Drawing for the job (mm, zero at the part's lowest x, y, z). Coordinates: 2 decimals unless noted, no trailing zeros. Write each loop counter-clockwise with the first axis right and the second up, starting at its lowest first coordinate (ties: lowest second). Pieces come first, ordered by that corner, then holes. Notation, with made-up numbers: M 11.25,67.25 L 29.25,67.25 A24 cw 29.25,84.25 Z; hole C 49,77 d2. An arc over 180 degrees is marked long. Use CSV: the item, a comma, the result in double quotes. Start each with the question number.
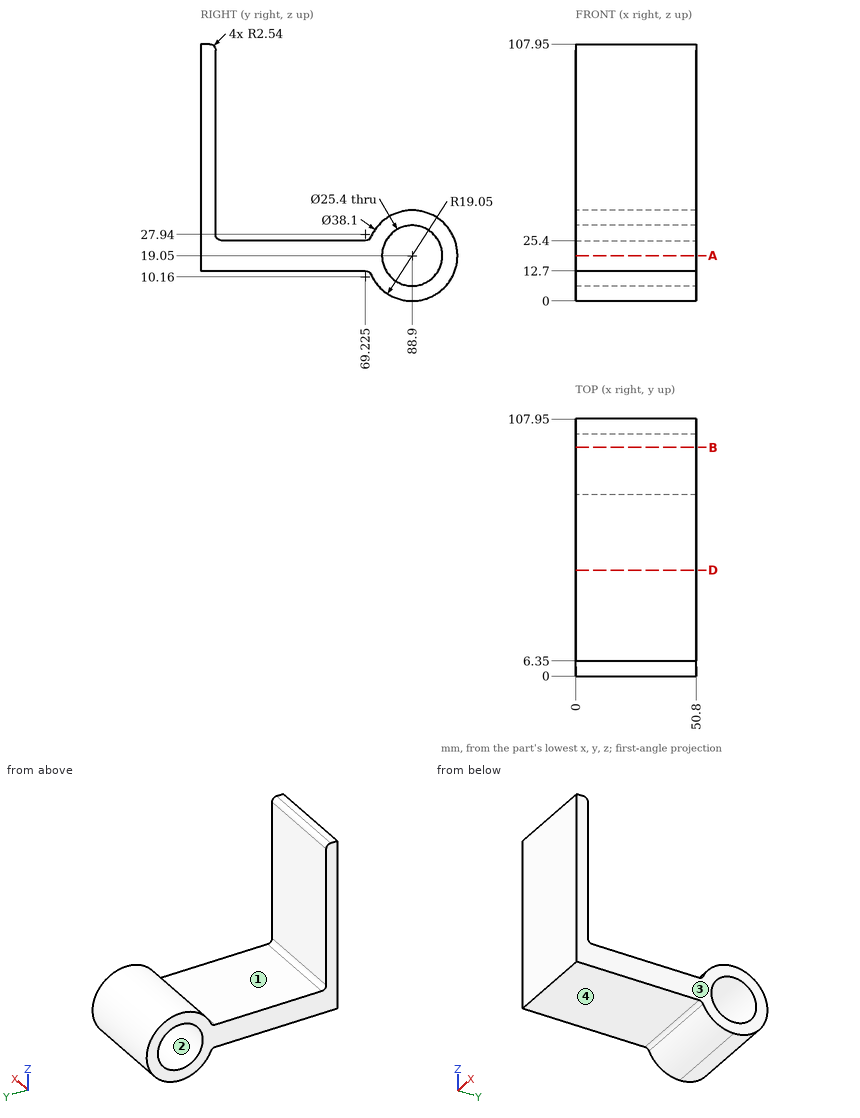
1) Band-saw the part on D-D on y = 44.5. List the corners of the cut face in (x, z), then the cut area to 3 significant figures.
2) Drop flat-ended pins along their axis: P1, Ø1.5, axis at x = 43, y = 47.5, coming from the -Z side; P2, Ø1, axis at x = 29, z = 92.5, coming from the +Y side; P3, Ø8, axis at x = 22, y = 56.5, coming from the +Z side; P4, Ø23, axis at y = 88.9, z = 19.05, coming from the +X side. Give the stop position or say it passes through.
3) Wall check: L1, parallel to Y at x = 35, z = 19.05; L2, parallel to Z at x = 15, y = 88; L3, parallel to Y at x = 12.5, z = 47.5. Give the ranges that are in metal, low to high. Write a range as [from, to].
4) Band-saw the part on A-A on z = 19.05. List the corners of the cut face in (x, y).
5) Band-saw the part on B-B on y = 96. List the corners of the cut face in (x, z).
6) Two-plate mould, pull along Z, no slides. Class the marked faces 1, 2, 3 and 4: pulls with the +Z half, pulls with the -Z half, needs draft (parallel to the pull), parting line crosses it, or undercut.
Findings below:
1,outline,"M 0,12.7 L 50.8,12.7 L 50.8,25.4 L 0,25.4 Z"
1,area,"645 mm2"
2,P1,"stops at z = 12.7"
2,P2,"stops at y = 6.35"
2,P3,"stops at z = 25.4"
2,P4,"passes through"
3,L1,"y = [0, 76.2], [101.6, 107.95]"
3,L2,"z = [0.02, 6.38], [31.72, 38.08]"
3,L3,"y = [0, 6.35]"
4,outline,"M 0,0 L 50.8,0 L 50.8,76.2 L 0,76.2 Z; M 0,101.6 L 50.8,101.6 L 50.8,107.95 L 0,107.95 Z"
5,outline,"M 0,1.37 L 50.8,1.37 L 50.8,8.52 L 0,8.52 Z; M 0,29.58 L 50.8,29.58 L 50.8,36.73 L 0,36.73 Z"
6,face 1,"pulls with the +Z half"
6,face 2,"undercut"
6,face 3,"needs draft"
6,face 4,"pulls with the -Z half"
